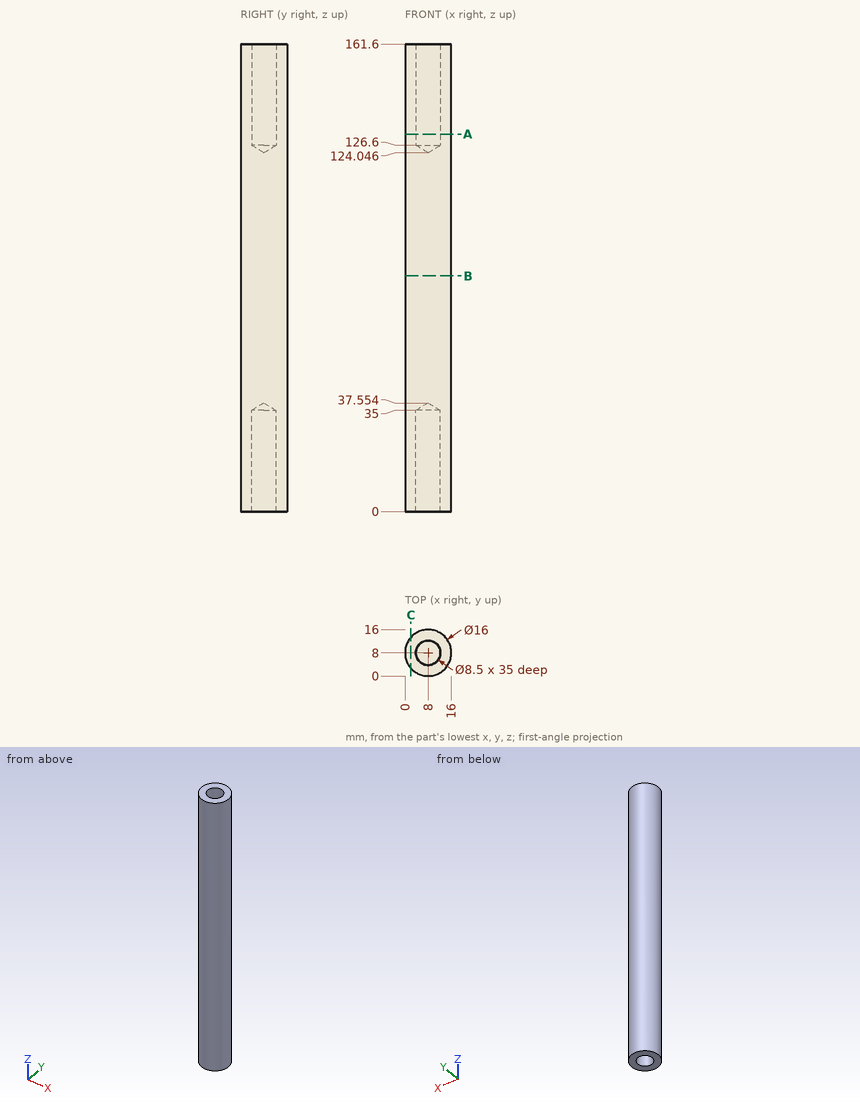
Verification items for this drawing (mm, ordinates from the low corner). Give positions to 0.01 mm unless a question says otherwise; leave off trailing zeros. Loops run counter-clockwise (first coordinate to the right, second up) from the corner with the lowest first, then second, coordinate; pieces in that order, holes last. Notation, with made-up numbers: M -35,60.5 L 17,60.5 A14 ccw 17,64.5 Z; hole C 27,-33 d9. An arc over 180 degrees is marked long. Answer in a Markdown table with one row per item.
1) Depth check by flat-ended pin: pin 1 (4 mm diameter, centred on x = 7.5, z = 28.5, fed in from +Y); pin 2 (5 mm diameter, centred on x = 8, y = 8, fed in from +Z); pin 3 (1.5 mm diameter, centred on x = 6, y = 10.5, fed in from -Z). Enter the tip coordinate at first touch or a pass-through.
Solutions:
| item | result |
|---|---|
| pin 1 | stops at y = 16 |
| pin 2 | stops at z = 125.55 |
| pin 3 | stops at z = 35.18 |
2) Thickness scan on line 1 (Y direction, x = 8, z = 23); line 2 (Y direction, x = 5.5, z = 130); line 3 (X direction, y = 11, z = 144) (1 decimal). Record the ranges inside material, lowest first.
Solutions:
| item | result |
|---|---|
| line 1 | y = 0 to 3.75, 12.25 to 16 |
| line 2 | y = 0.4 to 4.56, 11.44 to 15.6 |
| line 3 | x = 0.6 to 5, 11 to 15.4 |
3) Cross-section at C-C (x = 2). Enter the section's corners in (y, z), plus the area to 3 significant figures.
Solutions:
| item | result |
|---|---|
| outline | M 2.71,0 L 13.29,0 L 13.29,161.6 L 2.71,161.6 Z |
| area | 1,710 mm^2 |
4) Cross-section at B-B (z = 81.5). Enter the section's corners in (x, y), plus the area to 3 significant figures.
Solutions:
| item | result |
|---|---|
| outline | C 8,8 d16 |
| area | 201 mm^2 |
5) Cross-section at A-A (z = 130.5). Enter the section's corners in (x, y).
Solutions:
| item | result |
|---|---|
| outline | C 8,8 d16; hole C 8,8 d8.5 |
